Input: part model. Units: mm. Frame: model coordinates. Give positions to 0.01 mm unless a question says otherwise; leave off trailing zeros. Write each loop counter-clockwise with the first axis right and the second up, starting at its lowest first coordinate (ties: lowest second). Pieces come first, ordered by that corner, then holes. Notation, with made-up numbers: (17, -30) - (37, -30) arc R23 cw to (37, -3) - close; hole circle Ø6 at (52.5, 41.25). An arc over 180 degrees is marked (long way). Answer as CSV lines item,"result".
Autodesk Inventor part; units mm, degrees
ref_plane "YZ Plane" through (0, 0, 0) normal (1, 0, 0) x (0, 1, 0)
ref_plane "XZ Plane" through (0, 0, 0) normal (0, 1, 0) x (-1, 0, 0)
ref_plane "XY Plane" through (0, 0, 0) normal (0, 0, 1) x (1, 0, 0)
sketch "Boceto1" plane through (0, 0, 0) normal (0, 1, 0) x (-1, 0, 0)
  circle A0 centre (0, 0) radius 1
  dimension "d0" = 2
extrude "Extrusión1" add sketch "Boceto1" along normal mid plane 40.91
sketch "Boceto2" plane through (0, 20.455, 0) normal (0, 1, 0) x (1, 0, 0)
  circle A0 centre (0, 0) radius 1
  circle A1 centre (0, 0) radius 1
  line L0 (1, 0) -> (-1, 0)
revolve "Revolución1" add sketch "Boceto2" angle 360 about axis through (1, 20.455, 0) along (-1, 0, 0) picked at (0.2495, 0.221) contours L0 A0
sketch "Boceto3" plane through (0, -20.455, 0) normal (0, -1, 0) x (1, 0, 0)
  circle A0 centre (0, 0) radius 1
  circle A1 centre (0, 0) radius 1
  line L0 (1, 0) -> (-1, 0)
revolve "Revolución2" add sketch "Boceto3" angle 360 about axis through (1, -20.455, 0) along (-1, 0, 0) picked at (0.2495, 0.221) contours L0 A0
properties part number "EjeMotor"
Item 1: Contact query for a flat-ended pin moving along its axis: pin 1 (1 mm diameter, centred on x = -0.5, z = 0, fed in from -Y) (3 decimals). Output: stop coordinate, or through.
The answers:
pin 1,"y = -21.455"
Item 2: Cut plane C-C on z = -0.65. Return the cut outline in (x, y) (3 decimals).
The answers:
outline,"(-0.76, -20.455) arc R0.76 ccw to (0.76, -20.455) - (0.76, 20.455) arc R0.76 ccw to (-0.76, 20.455) - close"
Item 3: Cut plane B-B on x = 0.25. Return the cut outline in (y, z) (1 decimal), plus the area to 3 significant figures.
The answers:
outline,"(-20.5, -1) - (20.5, -1) arc R1 ccw to (20.5, 1) - (-20.5, 1) arc R1 ccw to start"
area,"82.2 mm²"
Item 4: Cut plane A-A on y = -14. Return the cut outline in (x, z), plus the area to 3 significant figures.
The answers:
outline,"circle Ø2 at (0, 0)"
area,"3.14 mm²"
Item 5: Ray query, line 1 (Z direction, x = 0.1, y = 10); line 2 (Z direction, x = 0.9, y = -13). Return the intervals inside material, ascending. Write a range as from..to.
The answers:
line 1,"-0.99..0.99"
line 2,"-0.44..0.44"
